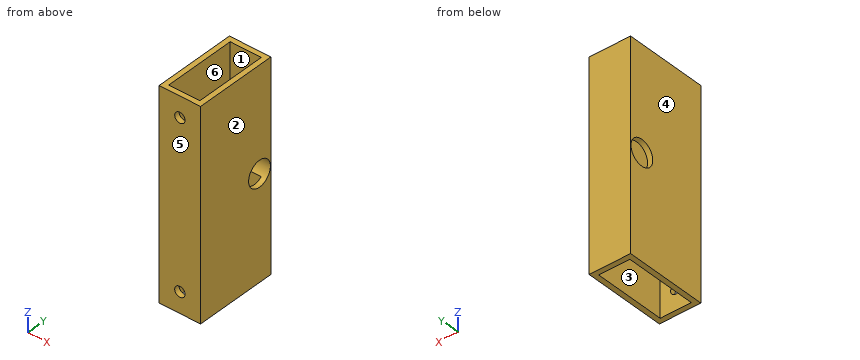
from build123d import *

# Parameters (mm, degrees)
SKETCH1_W           = 25.4
SKETCH1_H           = 50.8
SKETCH1_W_2         = 19.05
SKETCH1_H_2         = 44.45
BOSS_EXTRUDE1_DEPTH = 63.5
SKETCH2_R           = 7.874
CUT_EXTRUDE1_DEPTH  = 25.4
SKETCH3_R           = 3.175
CUT_EXTRUDE2_DEPTH  = 3.175


with BuildPart() as part:
    # Sketch1 → Boss-Extrude1 (new, symmetric)
    with BuildSketch(Plane.XY):
        with Locations((0.582385658, -5.091775964)):
            Rectangle(SKETCH1_W, SKETCH1_H)
        with Locations((0.582385658, -5.091775964)):
            Rectangle(SKETCH1_W_2, SKETCH1_H_2, mode=Mode.SUBTRACT)
    extrude(amount=BOSS_EXTRUDE1_DEPTH, both=True)

    # Sketch2 → Cut-Extrude1 (cut)
    with BuildSketch(Plane.ZY.offset(12.117614342)):
        with Locations(Location((0, 12.138059528, 0), (0, 0, 270))):
            Circle(SKETCH2_R)
    extrude(amount=-CUT_EXTRUDE1_DEPTH, mode=Mode.SUBTRACT)

    # Sketch3 → Cut-Extrude2 (cut)
    with BuildSketch(Plane.XZ.offset(30.491775964)):
        with Locations(Location((0.582385658, 50.8, 0), (0, 0, 270))):
            Circle(SKETCH3_R)
        with Locations(Location((0.582385658, -50.8, 0), (0, 0, 270))):
            Circle(SKETCH3_R)
    extrude(amount=-CUT_EXTRUDE2_DEPTH, mode=Mode.SUBTRACT)


solid = part.part
Source: CAD feature listing. Evaluate the final solid. Frame: model axes, mm. Face numbers are marked on the shaded views. A direction names the side the tool comes from. Give positions to 0.01 mm unless a question says otherwise; leave off trailing zeros. Write each loop counter-clockwise with the first axis right and the second up, starting at its lowest first coordinate (ties: lowest second). Pieces come first, ordered by that corner, then holes. Notation, with made-up numbers: M 64.25,2 L 105.25,2 A28 cw 105.25,38 Z; hole C -15.75,30.25 d1. An arc over 180 degrees is marked long. Return JSON: item names as keys, results as strings. Group by question number.
1) Cut plane A-A, the plane z = 0. Output: boundary loops of the cut face in (x, y), plus the area to 3 significant figures.
2) Pin query (flat end, axial travel): P1, Ø5, axis at x = 0.58, z = -50.8, coming from the -Y side. Return the tip coordinate at first contact, or that it passes through.
3) Pull-direction query (Y, two-part tool) for the marked faces 3, 4, 5 and 6; classes: pulls with the +Y half, pulls with the -Y half, needs draft (parallel to the pull), parting line crosses it, or undercut.
4) Cut plane B-B, the plane x = -5.25. Output: boundary loops of the cut face in (y, z), plus the area to 3 significant figures.
5) Set-up query: the marked faces 1 and 2. Return all of +Z, -Z, +X, -X, +Y, -Y with unobstructed straight access to the full face (end or side cutting, diameter ignored); none if empty.
6) Cut plane D-D, the plane z = -24. Output: boundary loops of the cut face in (x, y), plus the area to 3 significant figures.
7) Cut plane C-C, the plane y = -25. Output: boundary loops of the cut face in (x, z).
8) Material intervals for line 1 along Y through (x, z) = (-3.5, -8); line 2 along X through (y, z) = (-23, 44); line 3 along X through (y, z) = (-28.15, 50.8), sorted ascending. Write a range as [from, to].
Recorded:
{
 "1": {"outline": "M -12.12,-30.49 L 13.28,-30.49 L 13.28,4.26 L 10.11,4.26 L 10.11,-27.32 L -8.94,-27.32 L -8.94,4.26 L -12.12,4.26 Z; M -12.12,20.01 L 13.28,20.01 L 13.28,20.31 L -12.12,20.31 Z", "area": "289 mm²"},
 "2": {"P1": "stops at y = 17.13"},
 "3": {"face 3": "undercut", "face 4": "needs draft", "face 5": "pulls with the -Y half", "face 6": "undercut"},
 "4": {"outline": "M -30.49,-63.5 L -27.32,-63.5 L -27.32,63.5 L -30.49,63.5 Z; M 17.13,-63.5 L 20.31,-63.5 L 20.31,63.5 L 17.13,63.5 L 17.13,6.09 A7.87 cw 17.13,-6.09 Z", "area": "782 mm²"},
 "5": {"face 1": "+Z, -Z", "face 2": "+Z, -Z, +X, +Y, -Y"},
 "6": {"outline": "M -12.12,-30.49 L 13.28,-30.49 L 13.28,20.31 L -12.12,20.31 Z; hole M -8.94,-27.32 L 10.11,-27.32 L 10.11,17.13 L -8.94,17.13 Z", "area": "444 mm²"},
 "7": {"outline": "M -12.12,-63.5 L -8.94,-63.5 L -8.94,63.5 L -12.12,63.5 Z; M 10.11,-63.5 L 13.28,-63.5 L 13.28,63.5 L 10.11,63.5 Z"},
 "8": {"line 1": "y = [-30.49, -27.32], [17.13, 20.31]", "line 2": "x = [-12.12, -8.94], [10.11, 13.28]", "line 3": "x = [-12.12, -2.59], [3.76, 13.28]"}
}
